```python
from build123d import *

# Parameters (mm, degrees)
SKETCH_1_W            = 16
SKETCH_1_H            = 42
EXTRUDE_1_DEPTH       = 124
EXTRUDE_4_DEPTH       = 24.193161441
EXTRUDE_4_DEPTH_BACK  = 24.175019218
EXTRUDE_5_DEPTH       = 24.263214739
EXTRUDE_5_DEPTH_BACK  = 24.1979861
SKETCH_7_W            = 12
SKETCH_7_H            = 38
CUT_EXTRUDE_1_DEPTH   = 3
SKETCH_8_W            = 12
SKETCH_8_H            = 38
CUT_EXTRUDE_2_DEPTH   = 25
SKETCH_9_W            = 4
SKETCH_9_H            = 20
CUT_EXTRUDE_3_DEPTH   = 2
SKETCH_10_R           = 1.55
CUT_EXTRUDE_4_DEPTH   = 20
EXTRUDE_10_DEPTH      = 22.25
EXTRUDE_10_DEPTH_BACK = 22.25
SKETCH_13_W           = 70
SKETCH_13_H           = 18
CUT_EXTRUDE_5_DEPTH   = 22.25


with BuildPart() as part:
    # Эскиз1 → Бобышка-Вытянуть1 (new body)
    with BuildSketch(Plane.XY):
        Rectangle(SKETCH_1_W, SKETCH_1_H)
    extrude(amount=EXTRUDE_1_DEPTH)

    # Эскиз5 → Бобышка-Вытянуть4 (add, two sides: drawn at the far end of the back side and taken through both)
    with BuildSketch(Plane(origin=(0, 0, 0), x_dir=(1, 0, 0), z_dir=(0, 1, 0)).offset(-EXTRUDE_4_DEPTH_BACK)):
        with BuildLine():
            Line((-8, -37.48588549), (-8, -39.501953095))
            ThreePointArc((-8, -39.501953095), (0, -40), (8, -39.501953095))
            Line((8, -39.501953095), (8, -37.48588549))
            ThreePointArc((8, -37.48588549), (0, -38), (-8, -37.48588549))
        make_face()
    extrude(amount=EXTRUDE_4_DEPTH + EXTRUDE_4_DEPTH_BACK)

    # Эскиз6 → Бобышка-Вытянуть5 (add, two sides: drawn at the far end of the back side and taken through both)
    with BuildSketch(Plane(origin=(0, 0, 0), x_dir=(1, 0, 0), z_dir=(0, 1, 0)).offset(-EXTRUDE_5_DEPTH_BACK)):
        Polygon((-8, -57.5), (8, -65.5), (8, -67.736067977), (-8, -59.736067977), align=None)
    extrude(amount=EXTRUDE_5_DEPTH + EXTRUDE_5_DEPTH_BACK)

    # Эскиз7 → Вырез-Вытянуть1 (cut)
    with BuildSketch(Plane.XY.offset(124)):
        Rectangle(SKETCH_7_W, SKETCH_7_H)
    extrude(amount=-CUT_EXTRUDE_1_DEPTH, mode=Mode.SUBTRACT)

    # Эскиз8 → Вырез-Вытянуть2 (cut)
    with BuildSketch(Plane(origin=(0, 0, 0), x_dir=(-1, 0, 0), z_dir=(0, 0, -1))):
        Rectangle(SKETCH_8_W, SKETCH_8_H)
    extrude(amount=-CUT_EXTRUDE_2_DEPTH, mode=Mode.SUBTRACT)

    # Эскиз9 → Вырез-Вытянуть3 (cut)
    with BuildSketch(Plane.ZY.offset(8)):
        with Locations((23, 0)):
            Rectangle(SKETCH_9_W, SKETCH_9_H)
    extrude(amount=-CUT_EXTRUDE_3_DEPTH, mode=Mode.SUBTRACT)

    # Эскиз10 → Вырез-Вытянуть4 (cut)
    with BuildSketch(Plane.XY.offset(121)):
        with Locations((0, 10)):
            Circle(SKETCH_10_R)
        with Locations((0, -10)):
            Circle(SKETCH_10_R)
    extrude(amount=-CUT_EXTRUDE_4_DEPTH, mode=Mode.SUBTRACT)

    # Эскиз12 → Бобышка-Вытянуть10 (add, two sides: drawn at the far end of the back side and taken through both)
    with BuildSketch(Plane(origin=(0, 0, 0), x_dir=(1, 0, 0), z_dir=(0, 1, 0)).offset(-EXTRUDE_10_DEPTH_BACK)):
        Polygon((-8, -57.5), (8, -65.5), (8, -47.5019531), (8, -39.501953095), (-8, -39.501953095), align=None)
    extrude(amount=EXTRUDE_10_DEPTH + EXTRUDE_10_DEPTH_BACK)

    # Эскиз13 → Вырез-Вытянуть5 (cut)
    with BuildSketch(Plane.ZY.offset(8)):
        with Locations((67, 0)):
            Rectangle(SKETCH_13_W, SKETCH_13_H)
    extrude(amount=-CUT_EXTRUDE_5_DEPTH, mode=Mode.SUBTRACT)


solid = part.part
```
Check sheet for the modelled part. Datum: model origin and axes. Units: mm. A direction names the side the tool comes from. Coordinates: 2 decimals unless noted, no trailing zeros. Order: outer loops, then holes, each group sorted by start corner. A loop starts at its lowest first (then second) coordinate and runs counter-clockwise, first axis right, second up. Notation, with made-up numbers: M 58,-16.75 L 101,-16.75 A29 cw 101,16.25 Z; hole C 67,82.25 d11. An arc over 180 degrees is marked long. Write each question's results on one line, items separated by ' | '. Start each with the question number.
1. Cross-section at B-B on y = -16. Record the cut outline in (x, z), and give its area (3 significant figures).
2. Cross-section at D-D on z = 11. Record the cut outline in (x, y), and give its area (3 significant figures).
3. Go/stop test with flat-tipped pins: P1, Ø9.5, axis at x = -3, z = 9.5, coming from the -Y side; P2, Ø3, axis at x = -1, z = 77, coming from the +Y side; P3, Ø8, axis at x = -4, z = 48, coming from the +Y side. Record where each tip stops, or that it passes through.
4. Material ranges on probe 1 along Y at (x, z) = (0, 109.5); probe 2 along Y at (x, z) = (0.75, 44.5); probe 3 along Z at (x, y) = (-3.25, -5), recorded low to high.
5. Mould release check, pull along Y, two halves, no side actions. Record for faces 6 (the face through (6, 0, 12)), 7 (the face through (0, 23, 38)), 8 (the face through (0, 24.193, 39)): +Y half, -Y half, draft (parallel to the pull), parting line (faces both ways), or undercut.
6. Access from +Z, -Z, +X, -X, +Y, -Y to the whole of each face (thin tool, end or side, straight path). Record for faces 1 (the face through (0, 24.263, 63)), 2 (the face through (0, -10, 101)), 3 (the face through (-0.112, -23.238, 61.444)), 4 (the face through (0, -19, 12)), 5 (the face through (0, 9, 67)).
7. Cross-section at A-A on z = 88. Record the cut outline in (x, y).
Checks:
1) outline: M -8,0 L -6,0 L -6,25 L 6,25 L 6,0 L 8,0 L 8,124 L 6,124 L 6,121 L -6,121 L -6,124 L -8,124 Z | area: 1,650 mm²
2) outline: M -8,-21 L 8,-21 L 8,21 L -8,21 Z; hole M -6,-19 L 6,-19 L 6,19 L -6,19 Z | area: 216 mm²
3) P1: stops at y = -21 | P2: stops at y = 21 | P3: stops at y = 22.25
4) probe 1: y = -21 to -11.55, -8.45 to 8.45, 11.55 to 21 | probe 2: y = -22.25 to -9, 9 to 22.25 | probe 3: z = 25 to 32, 102 to 121
5) face 6: undercut | face 7: draft | face 8: +Y half
6) face 1: +Z, -Z, +X, -X, +Y | face 2: +Z | face 3: +X, -Y | face 4: -Z | face 5: +X, -X
7) outline: M -8,-21 L 8,-21 L 8,-9 L -8,-9 Z; M -8,9 L 8,9 L 8,21 L -8,21 Z
